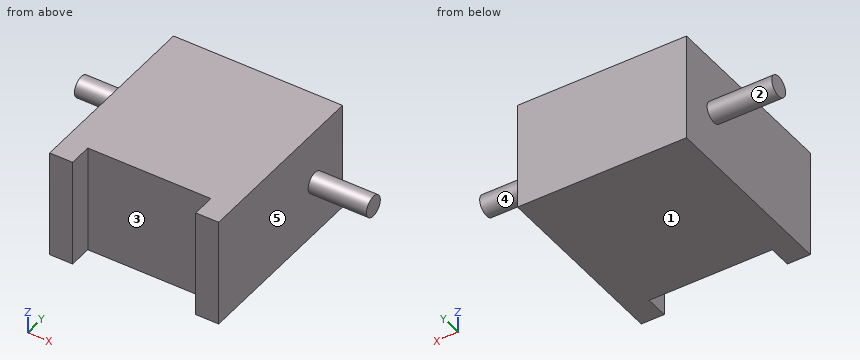
from build123d import *

# Parameters (mm, degrees)
SKETCH_1_W           = 40.5
SKETCH_1_H           = 45
EXTRUDE_1_DEPTH      = 26
SKETCH_2_W           = 29.5
SKETCH_2_H           = 5.5
CUT_EXTRUDE_1_DEPTH  = 38
EXTRUDE_2_DEPTH      = 14
EXTRUDE_2_DEPTH_BACK = 56
SKETCH_3_R           = 2.5


with BuildPart() as part:
    # 草图1 → 凸台-拉伸1 (new body)
    with BuildSketch(Plane.XY):
        with Locations((20.25, -22.5)):
            Rectangle(SKETCH_1_W, SKETCH_1_H)
    extrude(amount=EXTRUDE_1_DEPTH)

    # 草图2 → 切除-拉伸1 (cut)
    with BuildSketch(Plane.XY.offset(26)):
        with Locations((20.25, -42.25)):
            Rectangle(SKETCH_2_W, SKETCH_2_H)
    extrude(amount=-CUT_EXTRUDE_1_DEPTH, mode=Mode.SUBTRACT)

    # 草图3 → 凸台-拉伸2 (add, two sides: drawn at the far end of the back side and taken through both)
    with BuildSketch(Plane(origin=(40.5, 0, 0), x_dir=(0, 0, -1), z_dir=(1, 0, 0)).offset(-EXTRUDE_2_DEPTH_BACK)):
        with Locations((-13, -10)):
            Circle(SKETCH_3_R)
    extrude(amount=EXTRUDE_2_DEPTH + EXTRUDE_2_DEPTH_BACK)


solid = part.part
The listing builds one solid part. Answer for the finished solid, in the listing's coordinates (mm). Face numbers are marked on the shaded views. A direction names the side the tool comes from. Give positions to 0.01 mm unless a question says otherwise; leave off trailing zeros. Loops run counter-clockwise (first coordinate to the right, second up) from the corner with the lowest first, then second, coordinate; pieces in that order, holes last.
Item 1: Each of these flat-tipped pins is pushed along its axis until it touches: pin 1 Ø3 at (y, z) = (-14, 8.5) entering from +X; pin 2 Ø1.5 at (x, y) = (46.5, -12.5) entering from -Z; pin 3 Ø3 at (y, z) = (-41.5, 15.5) entering from -X; pin 4 Ø4 at (x, z) = (44, 3) entering from +Y (3 decimals). Where does it stop, or does it pass through?
Derived:
pin 1: stops at x = 40.5
pin 2: stops at z = 11.21
pin 3: stops at x = 0
pin 4: passes through
Item 2: A cutting plane is placed at B-B (y = -10). Give the vertices of the cut face in (x, z).
Derived:
outline: (-15.5, 10.5) - (0, 10.5) - (0, 0) - (40.5, 0) - (40.5, 10.5) - (54.5, 10.5) - (54.5, 15.5) - (40.5, 15.5) - (40.5, 26) - (0, 26) - (0, 15.5) - (-15.5, 15.5) - close
Item 3: A tool of negligible diameter and unlimited length cuts with its end or side. For the marked faces 1 and 2, from which of +Z, -Z, +X, -X, +Y, -Y can it reach the whole face along a straight path? Write none if from no direction.
Derived:
face 1: -Z, +X, -X, +Y, -Y
face 2: -X
Item 4: Find the intervals of material crossed by line 1 along X through (y, z) = (-33.5, 21.5); line 2 along Y through (x, z) = (23, 15.5); line 3 along Z through (x, y) = (-5.5, -10), in increasing order.
Derived:
line 1: x = 0 to 40.5
line 2: y = -39.5 to 0
line 3: z = 10.5 to 15.5
Item 5: A cutting plane is placed at D-D (z = 7). Give the vertices of the cut face in (x, y).
Derived:
outline: (0, -45) - (5.5, -45) - (5.5, -39.5) - (35, -39.5) - (35, -45) - (40.5, -45) - (40.5, 0) - (0, 0) - close
Item 6: Determine the mould class of the marked faces 3, 4 and 5 for opening direction X: +X half, -X half, draft (parallel to the pull), parting line (faces both ways), or undercut.
Derived:
face 3: undercut
face 4: draft
face 5: +X half
Item 7: A cutting plane is placed at C-C (x = 47.5). Give the vertices of the cut face in (y, z).
Derived:
outline: circle Ø5 at (-10, 13)
Item 8: A cutting plane is placed at A-A (z = 13). Give the vertices of the cut face in (x, y).
Derived:
outline: (-15.5, -12.5) - (0, -12.5) - (0, -45) - (5.5, -45) - (5.5, -39.5) - (35, -39.5) - (35, -45) - (40.5, -45) - (40.5, -12.5) - (54.5, -12.5) - (54.5, -7.5) - (40.5, -7.5) - (40.5, 0) - (0, 0) - (0, -7.5) - (-15.5, -7.5) - close
